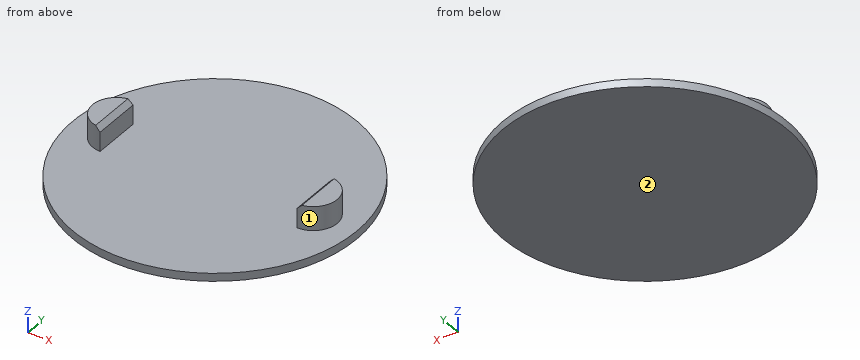
from build123d import *

# Parameters (mm, degrees)
F0_R     = 8.875
F1_DEPTH = 0.5
F3_DEPTH = 1.5
F4_SIZE  = 0.3


with BuildPart() as f1:
    # F0 (on Top) → F1 (new body)
    with BuildSketch(Plane.XY):
        Circle(F0_R)
    extrude(amount=F1_DEPTH)

    # F2 (on face) → F3 (join)
    with BuildSketch(Plane.XY.offset(0.5)):
        with BuildLine():
            Line((-6.15, -1.5), (-6.15, 1.5))
            ThreePointArc((-6.15, 1.5), (-7.65, 0), (-6.15, -1.5))
        make_face()
        with BuildLine():
            ThreePointArc((6.15, -1.5), (7.65, 0), (6.15, 1.5))
            Line((6.15, 1.5), (6.15, -1.5))
        make_face()
    extrude(amount=F3_DEPTH)

    # F4
    f4_edges = [f1.edges().sort_by_distance(p)[0] for p in [
        (-6.15, 0, 2),
        (6.15, 0, 2),
    ]]
    chamfer(f4_edges, length=F4_SIZE)


solid = f1.part
Geometry: final body of the model. Coordinates: model frame, mm. Face numbers are marked on the shaded views. A direction names the side the tool comes from. Coordinates: 2 decimals unless noted, no trailing zeros. Loops run counter-clockwise (first coordinate to the right, second up) from the corner with the lowest first, then second, coordinate; pieces in that order, holes last. Notation, with made-up numbers: (84.25, -33.5) - (122.25, -33.5) arc R22 ccw to (122.25, -1.5) - close; hole circle Ø8 at (-22.5, 15). An arc over 180 degrees is marked (long way). Put each result on its own line as item: value. Start each with the question number.
Q1. Line query: line 1 (Z direction, x = -4.25, y = 5); line 2 (Y direction, x = -6.5, z = 1.55); line 3 (Y direction, x = 3.75, z = 0.25). Output: solid intervals per line, ascending.
Q2. Cut plane A-A, the plane y = 0. Return loops of the section in (x, z) (3 decimals).
Q3. Cut plane B-B, the plane z = 0.9. Return loops of the section in (x, y).
Q4. Cut plane C-C, the plane x = 0. Return loops of the section in (y, z) (3 decimals).
Q5. Pin query (flat end, axial travel): pin 1 Ø3 at (x, y) = (-2.5, 5) entering from +Z; pin 2 Ø9 at (x, y) = (-3, 3.5) entering from +Z. Return the tip coordinate at first contact, or that it passes through.
Q6. Set-up query: the marked faces 1 and 2. Return all of +Z, -Z, +X, -X, +Y, -Y with unobstructed straight access to the full face (end or side cutting, diameter ignored); none if empty.
Q7. Cut plane D-D, the plane x = 5.25. Return loops of the section in (y, z), and give its area (3 significant figures).
Filled sheet:
1. line 1: 0 to 0.5
1. line 2: -1.46 to 1.46
1. line 3: -8.04 to 8.04
2. outline: (-8.875, 0) - (8.875, 0) - (8.875, 0.5) - (7.65, 0.5) - (7.65, 2) - (6.45, 2) - (6.15, 1.7) - (6.15, 0.5) - (-6.15, 0.5) - (-6.15, 1.7) - (-6.45, 2) - (-7.65, 2) - (-7.65, 0.5) - (-8.875, 0.5) - close
3. outline: (-6.15, -1.5) - (-6.15, 1.5) arc R1.5 ccw to start; (6.15, -1.5) arc R1.5 ccw to (6.15, 1.5) - close
4. outline: (-8.875, 0) - (8.875, 0) - (8.875, 0.5) - (-8.875, 0.5) - close
5. pin 1: z = 0.5
5. pin 2: z = 2
6. face 1: +Z, +X
6. face 2: -Z, +X, -X, +Y, -Y
7. outline: (-7.16, 0) - (7.16, 0) - (7.16, 0.5) - (-7.16, 0.5) - close
7. area: 7.16 mm²
